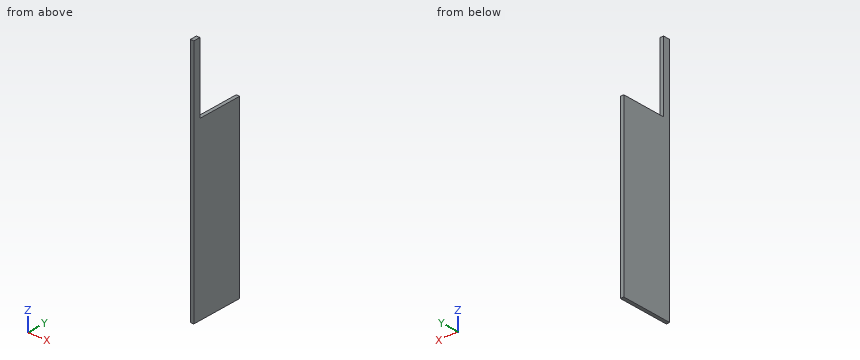
```python
from build123d import *

# Parameters (mm, degrees)
CROQUIS1_W              = 20
CROQUIS1_H              = 2
CROQUIS1_W_2            = 50
CROQUIS1_H_2            = 15
SALIENTE_EXTRUIR1_DEPTH = 1


with BuildPart() as part:
    # Croquis1 → Saliente-Extruir1 (new body)
    with BuildSketch(Plane(origin=(0, 0, 0), x_dir=(0, 0, -1), z_dir=(1, 0, 0))):
        with Locations((-35, -6.5)):
            Rectangle(CROQUIS1_W, CROQUIS1_H)
        Rectangle(CROQUIS1_W_2, CROQUIS1_H_2)
    extrude(amount=SALIENTE_EXTRUIR1_DEPTH)


solid = part.part
```
Geometry check sheet. Reference: the model listing, model coordinates, mm. Give positions to 0.01 mm unless a question says otherwise; leave off trailing zeros. Loops run counter-clockwise (first coordinate to the right, second up) from the corner with the lowest first, then second, coordinate; pieces in that order, holes last. Notation, with made-up numbers: M 83.5,78.5 L 108.5,78.5 A36 cw 108.5,112.5 Z; hole C -39,80 d11. An arc over 180 degrees is marked long. Write item = value, one per line.
(1) Sectioned sample at A-A, the plane z = 37.5. Record the cut outline in (x, y).
Answer below:
outline = M 0,-7.5 L 1,-7.5 L 1,-5.5 L 0,-5.5 Z
(2) Material ranges on line 1 (Z direction, x = 0.5, y = 3); line 2 (Y direction, x = 0.55, z = 40), recorded low to high. Write a range as [from, to].
Answer below:
line_1 = [-25, 25]
line_2 = [-7.5, -5.5]
(3) Sectioned sample at C-C, the plane x = 0.2. Record the cut outline in (y, z).
Answer below:
outline = M -7.5,-25 L 7.5,-25 L 7.5,25 L -5.5,25 L -5.5,45 L -7.5,45 Z
(4) Sectioned sample at B-B, the plane y = 1.25. Record the cut outline in (x, z), plus the area to 3 significant figures.
Answer below:
outline = M 0,-25 L 1,-25 L 1,25 L 0,25 Z
area = 50.0 mm2
